Geometry check sheet. Reference: the model listing, model coordinates, mm. Coordinates: 2 decimals unless noted, no trailing zeros. Order: outer loops, then holes, each group sorted by start corner. A loop starts at its lowest first (then second) coordinate and runs counter-clockwise, first axis right, second up.
```python
from build123d import *

# Parameters (mm, degrees)
CUT_EXTRUDE1_START = -250
SKETCH3_R          = 50
CUT_EXTRUDE1_DEPTH = 250


with BuildPart() as part:
    # Sketch2 → Revolve1 (revolve)
    with BuildSketch(Plane(origin=(0, 0, 0), x_dir=(0, 0, -1), z_dir=(1, 0, 0)), mode=Mode.PRIVATE) as revolve1_sk:
        Polygon((0, 0), (0, 50), (426.2, 50), (426.2, 37.5), (451.2, 37.5), (451.2, 50), (536, 50), (536, 37.5), (561, 37.5), (561, 50), (700, 50), (700, 0), align=None)
    revolve(revolve1_sk.sketch.rotate(Axis((0, 0, 0), (0, 0, -1)), 90), axis=Axis((0, 0, 0), (0, 0, -1)))

    # Sketch3 → Cut-Extrude1 (cut)
    with BuildSketch(Plane.XY.offset(CUT_EXTRUDE1_START)):
        Circle(SKETCH3_R)
    extrude(amount=CUT_EXTRUDE1_DEPTH, mode=Mode.SUBTRACT)


solid = part.part
```
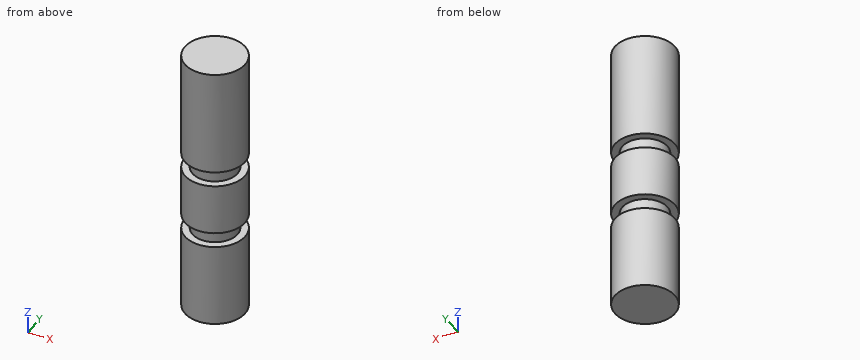
Item 1: Sectioned sample at C-C (x = -41.5). Record the cut outline in (y, z), and give its area (3 significant figures).
Item 2: Depth check by flat-ended pin: P1, Ø5, axis at y = 3.5, z = -508.5, coming from the -X side; P2, Ø8, axis at x = -26.5, z = -560.5, coming from the -Y side; P3, Ø12, axis at y = -22.5, z = -394.5, coming from the -X side. Enter the tip coordinate at first touch or a pass-through.
Item 3: Sectioned sample at A-A (x = 0). Record the cut outline in (y, z), and give its area (4 significant figures).
Item 4: Thickness scan on line 1 along Z through (x, y) = (36.5, 25); line 2 along Y through (x, z) = (1, -520.5); line 3 along X through (y, z) = (-10.5, -482). Record the ranges inside material, lowest first.
Item 5: Sectioned sample at B-B (y = -43). Record the cut outline in (x, z).
Geometry check:
1. outline: (-27.89, -700) - (27.89, -700) - (27.89, -561) - (-27.89, -561) - close; (-27.89, -536) - (27.89, -536) - (27.89, -451.2) - (-27.89, -451.2) - close; (-27.89, -426.2) - (27.89, -426.2) - (27.89, -250) - (-27.89, -250) - close
1. area: 22,300 mm2
2. P1: stops at x = -49.99
2. P2: stops at y = -44.64
2. P3: stops at x = -47.2
3. outline: (-50, -700) - (50, -700) - (50, -561) - (37.5, -561) - (37.5, -536) - (50, -536) - (50, -451.2) - (37.5, -451.2) - (37.5, -426.2) - (50, -426.2) - (50, -250) - (-50, -250) - (-50, -426.2) - (-37.5, -426.2) - (-37.5, -451.2) - (-50, -451.2) - (-50, -536) - (-37.5, -536) - (-37.5, -561) - (-50, -561) - close
3. area: 43,750 mm2
4. line 1: z = -700 to -561, -536 to -451.2, -426.2 to -250
4. line 2: y = -49.99 to 49.99
4. line 3: x = -48.89 to 48.89
5. outline: (-25.51, -700) - (25.51, -700) - (25.51, -561) - (-25.51, -561) - close; (-25.51, -536) - (25.51, -536) - (25.51, -451.2) - (-25.51, -451.2) - close; (-25.51, -426.2) - (25.51, -426.2) - (25.51, -250) - (-25.51, -250) - close
